Input: dimensioned drawing with shaded views. Units: mm. Origin: part minimum x, y, z. Give positions to 0.01 mm unless a question says otherwise; leave off trailing zeros. Order: outer loops, then holes, each group sorted by start corner. A loop starts at its lowest first (then second) coordinate and runs counter-clockwise, first axis right, second up.
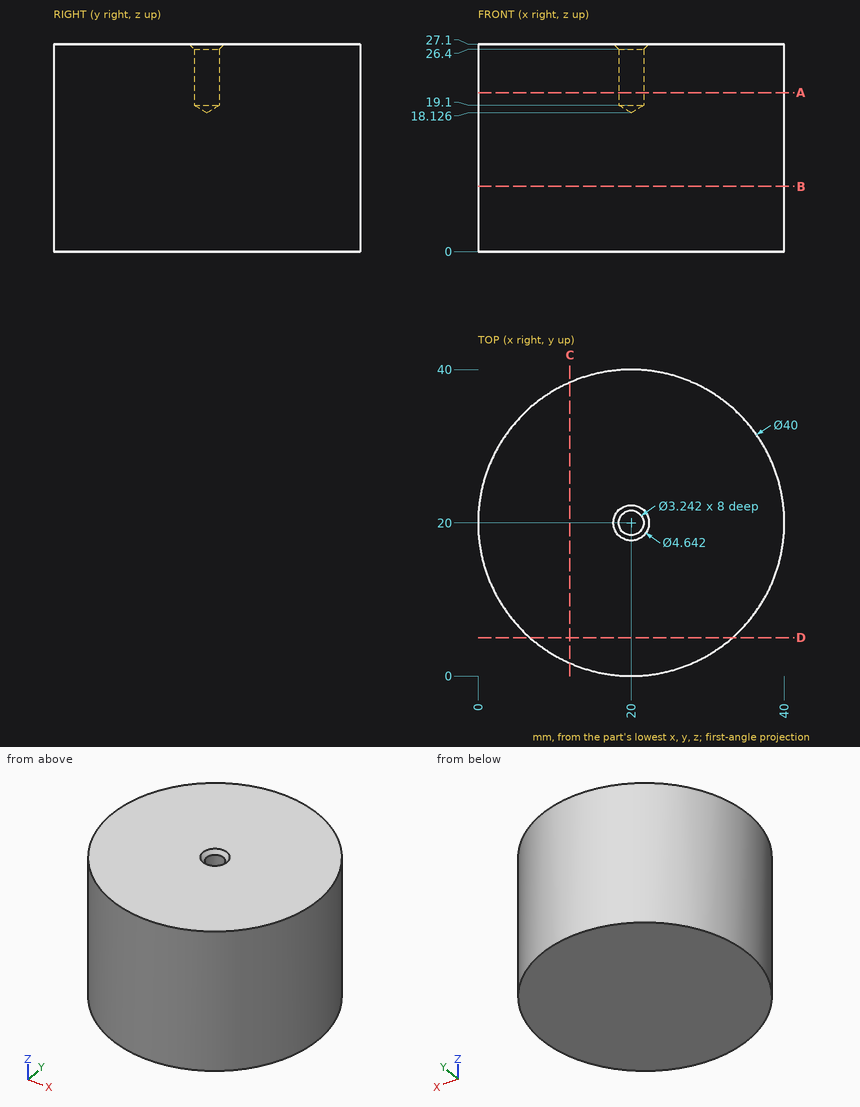
1) Section query B-B, the plane z = 8.5. Return the cut outline in (x, y).
Report:
outline: circle Ø40 at (20, 20)
2) Pin query (flat end, axial travel): pin 1 (3 mm diameter, centred on y = 7, z = 3, fed in from -X); pin 2 (5 mm diameter, centred on y = 23.5, z = 21.5, fed in from +X) (3 decimals); pin 3 (8 mm diameter, centred on x = 27, z = 9, fed in from +Y). Return the tip coordinate at first contact, or that it passes through.
Report:
pin 1: stops at x = 3.64
pin 2: stops at x = 39.975
pin 3: stops at y = 39.77
3) Material intervals for L1, parallel to Y at x = 20, z = 20.75; L2, parallel to X at y = 37, z = 9; L3, parallel to Y at x = 7, z = 4.75, sorted ascending.
Report:
L1: y = 0 to 18.38, 21.62 to 40
L2: x = 9.46 to 30.54
L3: y = 4.8 to 35.2
4) Section query C-C, the plane x = 12. Return the cut outline in (y, z).
Report:
outline: (1.67, 0) - (38.33, 0) - (38.33, 27.1) - (1.67, 27.1) - close
5) Section query D-D, the plane y = 5. Return the cut outline in (x, z).
Report:
outline: (6.77, 0) - (33.23, 0) - (33.23, 27.1) - (6.77, 27.1) - close
6) Section query A-A, the plane z = 20.75. Return the cut outline in (x, y), and give its area (3 significant figures).
Report:
outline: circle Ø40 at (20, 20); hole circle Ø3.24 at (20, 20)
area: 1,250 mm2
